from build123d import *

# Parameters (mm, degrees)
CHAMFER_1_SIZE = 0.5


with BuildPart() as part:
    # Эскиз1 → Повернуть1 (revolve)
    with BuildSketch(Plane.XY):
        Polygon((0, 0), (-5, 0), (-5, 15), (-6, 15), (-6, 54), (-8, 54), (-8, 738), (-5, 738), (-5, 746), (-4.8, 746), (-4.8, 747.15), (-5, 747.15), (-5, 750), (0, 750), align=None)
    revolve(axis=Axis((0, 750, 0), (0, -1, 0)))

    # Фаска1
    chamfer_1_edges = [part.edges().sort_by_distance(p)[0] for p in [
        (8, 738, 0),
        (8, 54, 0),
        (6, 15, 0),
        (5, 0, 0),
        (5, 750, 0),
    ]]
    chamfer(chamfer_1_edges, length=CHAMFER_1_SIZE)


solid = part.part
For this review, take the finished solid that the model builds, in its own axes (mm). A direction names the side the tool comes from. Coordinates: 2 decimals unless noted, no trailing zeros. Loops run counter-clockwise (first coordinate to the right, second up) from the corner with the lowest first, then second, coordinate; pieces in that order, holes last. Notation, with made-up numbers: (68.25, 37.5) - (95.25, 37.5) arc R29 ccw to (95.25, 76.5) - close; hole circle Ø2 at (-29, -31). An arc over 180 degrees is marked (long way). Return JSON: item names as keys, results as strings.
Item 1: For faces 1 (the cylindrical face through (1.73, 400.78, 7.81)), 2 (the flat face through (-2, 738, 5)), 3 (the flat face through (2, 54, -6)), list the 3-axis set-ups (+Z, -Z, +X, -X, +Y, -Y) from which the entire face can be reached by the end or side of a thin tool; tool diameter is ignored.
Determined:
{"face 1": "+Y, -Y", "face 2": "+Y", "face 3": "-Y"}
Item 2: Take a section at C-C (y = 500.5). Give the boundary of the cut face in (x, z), then the cut area to 3 significant figures.
Determined:
{"outline": "circle Ø16 at (0, 0)", "area": "201 mm2"}
Item 3: For line 1 (Z direction, x = 6.25, y = 684); line 2 (X direction, y = 491.5, z = 0.5); line 3 (Z direction, x = 1.5, y = 660), list the stretches that pass through material, from the lowest coordinate up.
Determined:
{"line 1": "z = -4.99 to 4.99", "line 2": "x = -7.98 to 7.98", "line 3": "z = -7.86 to 7.86"}
Item 4: Insertion check: pin 1 (8 mm diameter, centred on y = 249.5, z = 5.5, fed in from +X); pin 2 (1.5 mm diameter, centred on x = -3, y = 656.5, fed in from -Z); pin 3 (5 mm diameter, centred on y = 103.5, z = 5.5, fed in from +X). Each pin has a flat end and moves straight along its axis. Give the tip position at first contact, or say it passes through.
Determined:
{"pin 1": "stops at x = 7.86", "pin 2": "stops at z = -7.68", "pin 3": "stops at x = 7.42"}
